Geometry: final body of the model. Coordinates: model frame, mm. A direction names the side the tool comes from. Give positions to 0.01 mm unless a question says otherwise; leave off trailing zeros. Loops run counter-clockwise (first coordinate to the right, second up) from the corner with the lowest first, then second, coordinate; pieces in that order, holes last. Notation, with made-up numbers: (17.5, 18) - (47.5, 18) arc R13 cw to (47.5, 39) - close; hole circle Ø8 at (32.25, 78.5). An arc over 180 degrees is marked (long way). Use CSV: the item, a comma, the result in double quotes. Start each with the question number.
```python
from build123d import *

# Parameters (mm, degrees)
F0_W     = 38.054697
F0_H     = 19.05
F1_DEPTH = 6.35
F2_W     = 25.4
F2_H     = 6.35
F3_DEPTH = 38.1
F4_W     = 25.4
F4_H     = 25.4
F5_DEPTH = 12.7


with BuildPart() as f1:
    # F0 (on Front) → F1 (new body)
    with BuildSketch(Plane.XZ):
        with Locations((19.027348, 9.525)):
            Rectangle(F0_W, F0_H)
    extrude(amount=F1_DEPTH)

    # F2 (on Right) → F3 (join)
    with BuildSketch(Plane.YZ):
        with Locations((-12.7, 3.175)):
            Rectangle(F2_W, F2_H)
    extrude(amount=F3_DEPTH)

    # F4 (on Right) → F5 (join)
    with BuildSketch(Plane.YZ):
        with Locations((-12.7, 12.7)):
            Rectangle(F4_W, F4_H)
    extrude(amount=F5_DEPTH)


solid = f1.part
```
Item 1: Ray query, probe 1 along X at (y, z) = (-14.25, 24); probe 2 along Y at (x, z) = (22.5, 16.5); probe 3 along Z at (x, y) = (14, -16.5). Return the intervals inside material, ascending.
Item 2: Section A-A (z = 15). Output: boundary loops of the cut face in (x, y).
Item 3: Reachability of faces 1 (the flat face through (25, -6.35, 13)), 2 (the flat face through (25, -3, 19.05)), 3 (the flat face through (19, 0, 10)) from +Z, -Z, +X, -X, +Y, -Y: full face, straight path, thin tool, end or side. Return the list, or none.
Item 4: Section B-B (y = -2.5). Output: boundary loops of the cut face in (x, z), plus the area to 3 significant figures.
Item 5: Pin query (flat end, axial travel): pin 1 Ø1.5 at (y, z) = (-21, 13) entering from +X; pin 2 Ø4 at (x, z) = (26.5, 15) entering from -Y; pin 3 Ø5 at (y, z) = (-3.5, 14.5) entering from +X. Return the tip coordinate at first contact, or that it passes through.
Item 6: Section D-D (y = -11.25). Output: boundary loops of the cut face in (x, z).
Item 7: Section C-C (x = 21). Output: boundary loops of the cut face in (y, z).
Outcome:
1,probe 1,"x = 0 to 12.7"
1,probe 2,"y = -6.35 to 0"
1,probe 3,"z = 0 to 6.35"
2,outline,"(0, -25.4) - (12.7, -25.4) - (12.7, -6.35) - (38.05, -6.35) - (38.05, 0) - (0, 0) - close"
3,face 1,"+Z, +X, -Y"
3,face 2,"+Z, +X, +Y, -Y"
3,face 3,"+Z, -Z, +X, -X, +Y"
4,outline,"(0, 0) - (38.1, 0) - (38.1, 6.35) - (38.05, 6.35) - (38.05, 19.05) - (12.7, 19.05) - (12.7, 25.4) - (0, 25.4) - close"
4,area,"806 mm2"
5,pin 1,"stops at x = 12.7"
5,pin 2,"stops at y = -6.35"
5,pin 3,"stops at x = 38.05"
6,outline,"(0, 0) - (38.1, 0) - (38.1, 6.35) - (12.7, 6.35) - (12.7, 25.4) - (0, 25.4) - close"
7,outline,"(-25.4, 0) - (0, 0) - (0, 19.05) - (-6.35, 19.05) - (-6.35, 6.35) - (-25.4, 6.35) - close"
